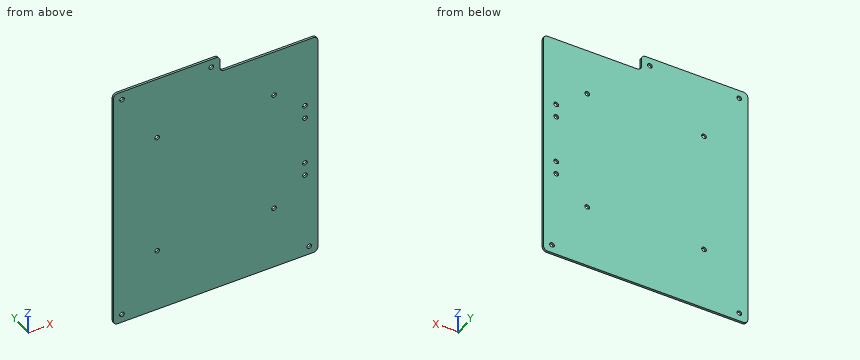
Autodesk Inventor part; units mm, degrees
ref_plane "YZ Plane" through (0, 0, 0) normal (1, 0, 0) x (0, 1, 0)
ref_plane "XZ Plane" through (0, 0, 0) normal (0, 1, 0) x (-1, 0, 0)
ref_plane "XY Plane" through (0, 0, 0) normal (0, 0, 1) x (1, 0, 0)
sketch "Sketch1" plane through (0, 0, 0) normal (0, 1, 0) x (-1, 0, 0)
  line L0 (50.4698, -94.8182) -> (63.1698, -94.8182)
  line L1 (63.1698, -94.8182) -> (63.1698, -82.1182)
  line L2 (50.4698, 94.8182) -> (63.1698, 94.8182)
  line L3 (63.1698, 94.8182) -> (63.1698, 82.1182)
  circle A0 centre (56.8198, 88.4682) radius 1.75
  circle A1 centre (56.8198, -88.4682) radius 1.75
  circle A2 centre (-82.2198, -88.4682) radius 1.75
  line L4 (-15.875, 82.1182) -> (-15.875, 94.8182)
  line L5 (-15.875, 94.8182) -> (-3.175, 94.8182)
  circle A3 centre (-9.525, 88.4682) radius 1.75
  line L6 (-15.875, 94.8182) -> (63.1698, 94.8182)
  line L7 (63.1698, 94.8182) -> (63.1698, -94.8182)
  line L8 (63.1698, -94.8182) -> (-88.5698, -94.8182)
  line L9 (-15.875, 82.1182) -> (-88.5698, 82.1182)
  line L10 (-88.5698, -94.8182) -> (-88.5698, 82.1182)
  circle A4 centre (-56.047, -46.609) radius 1.75
  circle A5 centre (-56.047, -46.609) radius 1.75
  circle A6 centre (30.647, -46.609) radius 1.75
  circle A7 centre (30.647, -46.609) radius 1.75
  circle A8 centre (30.647, 46.609) radius 1.75
  circle A9 centre (30.647, 46.609) radius 1.75
  circle A10 centre (-56.047, 46.609) radius 1.75
  circle A11 centre (-56.047, 46.609) radius 1.75
  point P0 (15.9004, 85.2932)
  point P1 (63.1698, 85.2932)
  point P2 (63.1698, -85.2932)
extrude "Extrusion1" add sketch "Sketch1" along normal blind 1.5875
fillet "Fillet1" radius 3.175 6 edges at (-63.1698, 0.7937, 94.8182) (15.875, 0.7937, 94.8182) (15.875, 0.7937, 82.1182) (88.5698, 0.7937, 82.1182) (88.5698, 0.7937, -94.8182) (-63.1698, 0.7937, -94.8182)
sketch "Sketch2" plane through (0, 1.5875, 0) normal (0, 1, 0) x (1, 0, 0)
  line L0 (-63.1698, 91.6432) -> (-63.1698, -91.6432)
  arc A0 (-59.9948, 94.8182) -> (-63.1698, 91.6432) centre (-59.9948, 91.6432) ccw
  line L1 (-63.1698, 91.6432) -> (-63.1698, -91.6432)
  line L2 (88.5698, -78.9432) -> (88.5698, 91.6432)
  line L3 (69.5198, 0) -> (69.5198, -38.1)
  line L4 (69.5198, -38.1) -> (88.5698, -38.1)
  line L5 (88.5698, -38.1) -> (88.5698, 0)
  line L6 (88.5698, -38.1) -> (69.5198, -38.1)
  line L7 (69.5198, -38.1) -> (69.5198, 38.1)
  line L8 (69.5198, 38.1) -> (88.5698, 38.1)
  line L9 (88.5698, 38.1) -> (88.5698, -38.1)
  line L10 (69.5198, -38.1) -> (88.5698, -38.1)
  line L11 (88.5698, -38.1) -> (88.5698, -19.05)
  line L12 (69.5198, -19.05) -> (69.5198, -38.1)
  circle A1 centre (79.0448, -28.575) radius 1.75
  line L13 (69.5198, 38.1) -> (88.5698, 38.1)
  line L14 (88.5698, 38.1) -> (88.5698, 19.05)
  line L15 (69.5198, 19.05) -> (69.5198, 38.1)
  circle A2 centre (79.0448, 28.575) radius 1.75
  circle A3 centre (79.0448, -18.415) radius 1.75
  circle A4 centre (79.0448, 18.415) radius 1.75
  point P0 (0, 0)
  dimension "d3" = 19.05
  dimension "d7" = 19.05
  dimension "d8" = 3.5
  dimension "d9" = 19.05
  dimension "d10" = 3.5
  dimension "d15" = 3.5
  dimension "d16" = 3.5
extrude "Extrusion3" cut sketch "Sketch2" against normal blind 25.4 contours A1 | A2 | A3 | A4
properties part number "bottomMountingPlate2"
CAD build for the part. Positions are in the model's coordinates, mm. Coordinates: 2 decimals unless noted, no trailing zeros. Loops run counter-clockwise (first coordinate to the right, second up) from the corner with the lowest first, then second, coordinate; pieces in that order, holes last. Notation, with made-up numbers: (57.5, -25.5) - (75.5, -25.5) arc R21 ccw to (75.5, -10.5) - close; hole circle Ø10 at (12, 72.5). An arc over 180 degrees is marked (long way). Use one line per item in the form item = value. Start each with the question number.
1) Band-saw the part on B-B (x = 41.5). Give the cut face in (y, z).
2) Flat gauge pins, fed straight in: pin 1 (4 mm diameter, centred on x = -30.647, z = 46.609, fed in from -Y); pin 2 (0.8 mm diameter, centred on y = 1, z = 88.5, fed in from +X) (3 decimals). Where does each tip first touch, or does it go through?
3) Band-saw the part on A-A (y = 0.3). State how many separate pieces and enclosed holes the cut face has, and give its area (3 significant figures).
4) Drill centre lines: L1, parallel to Z at x = -31, y = 0.8; L2, parallel to Z at x = 63, y = 1.5; L3, parallel to Z at x = 55, y = 1.5. Where is each one in solid material? Low to high. Write a range as from..to.
Check values:
q1.outline = (0, -94.82) - (1.59, -94.82) - (1.59, 82.12) - (0, 82.12) - close
q2.pin_1 = 0
q2.pin_2 = 15.875
q3.separate_pieces = 1
q3.enclosed_holes = 12
q3.area = 27,700 mm2
q4.L1 = -94.82..-48.32, -44.89..44.89, 48.32..94.82
q4.L2 = -94.82..82.12
q4.L3 = -94.82..-48.01, -45.21..45.21, 48.01..82.12
